Design review of the part built by this model. Coordinates are the model's own, in mm. A direction names the side the tool comes from. Give positions to 0.01 mm unless a question says otherwise; leave off trailing zeros. Write each loop counter-clockwise with the first axis right and the second up, starting at its lowest first coordinate (ties: lowest second). Pieces come first, ordered by that corner, then holes.
```python
from build123d import *
from build123d.topology import SkipClean

# Parameters (mm, degrees)
SKETCH1_R           = 1.1
BOSS_EXTRUDE1_DEPTH = 1.12
SKETCH1_3_W         = 5.75
SKETCH1_3_H         = 5.75
BOSS_EXTRUDE2_DEPTH = 7
SKETCH1_4_W         = 10.8
SKETCH1_4_H         = 10.8
SKETCH1_4_W_2       = 5.75
SKETCH1_4_H_2       = 5.75
BOSS_EXTRUDE3_DEPTH = 5
BOSS_EXTRUDE4_DEPTH = 2
BOSS_EXTRUDE5_START = 0.1
SKETCH1_7_R         = 2
SKETCH1_7_R_2       = 1.1
BOSS_EXTRUDE5_DEPTH = 0.1
CHAMFER1_SIZE       = 1.7
SKETCH3_R           = 2.25
BOSS_EXTRUDE6_DEPTH = 1
BOSS_EXTRUDE6_TAPER = 60
FILLET1_R           = 1.5
SKETCH4_W           = 13
SKETCH4_H           = 4
BOSS_EXTRUDE7_DEPTH = 2.75


with BuildPart() as part:
    # Sketch1 → Boss-Extrude1 (new body)
    with BuildSketch(Plane(origin=(0, 0, 0), x_dir=(1, 0, 0), z_dir=(0, 1, 0))):
        with BuildLine():
            Line((-10.5, -11.931), (10.5, -11.931))
            ThreePointArc((10.5, -11.931), (11.914213562, -11.345213562), (12.5, -9.931))
            Line((12.5, -9.931), (12.5, 9.931))
            ThreePointArc((12.5, 9.931), (11.914213567, 11.345213558), (10.500000012, 11.931))
            Line((10.500000012, 11.931), (-10.5, 11.931))
            ThreePointArc((-10.5, 11.931), (-11.914213562, 11.345213562), (-12.5, 9.931))
            Line((-12.5, 9.931), (-12.5, -9.930999993))
            ThreePointArc((-12.5, -9.930999993), (-11.914213565, -11.34521356), (-10.5, -11.931))
        make_face()
        with Locations(Location((10.5, 2.769, 0), (0, 0, 270))):
            Circle(SKETCH1_R, mode=Mode.SUBTRACT)
        with Locations(Location((10.5, -9.931, 0), (0, 0, 270))):
            Circle(SKETCH1_R, mode=Mode.SUBTRACT)
        with Locations(Location((-10.5, -9.931, 0), (0, 0, 270))):
            Circle(SKETCH1_R, mode=Mode.SUBTRACT)
        with Locations(Location((-10.5, 2.769, 0), (0, 0, 270))):
            Circle(SKETCH1_R, mode=Mode.SUBTRACT)
    extrude(amount=-BOSS_EXTRUDE1_DEPTH)

    # Sketch1_3 → Boss-Extrude2 (add)
    with BuildSketch(Plane(origin=(0, 0, 0), x_dir=(1, 0, 0), z_dir=(0, 1, 0))):
        with Locations((0, 2.769)):
            Rectangle(SKETCH1_3_W, SKETCH1_3_H)
    extrude(amount=BOSS_EXTRUDE2_DEPTH)

    # Sketch1_4 → Boss-Extrude3 (add)
    with BuildSketch(Plane(origin=(0, 0, 0), x_dir=(1, 0, 0), z_dir=(0, 1, 0))):
        with Locations((0, 2.769)):
            Rectangle(SKETCH1_4_W, SKETCH1_4_H)
        with Locations((0, 2.769)):
            Rectangle(SKETCH1_4_W_2, SKETCH1_4_H_2, mode=Mode.SUBTRACT)
    extrude(amount=BOSS_EXTRUDE3_DEPTH)

    # Sketch1_6 → Boss-Extrude4 (add)
    with BuildSketch(Plane(origin=(0, 0, 0), x_dir=(1, 0, 0), z_dir=(0, 1, 0))):
        Polygon((3.5, -2.631), (-2.4, -2.631), (-2.4, -9.931), (6.5, -9.931), (6.5, -5.931), (3.5, -5.931), align=None)
    extrude(amount=BOSS_EXTRUDE4_DEPTH)

    # Sketch1_7 → Boss-Extrude5 (add)
    # profile 1 of 4: a face of its own
    with SkipClean():  # the faces are left unmerged after this step: merging them gives an invalid solid
        with BuildSketch(Plane(origin=(0, 0, 0), x_dir=(1, 0, 0), z_dir=(0, 1, 0)).offset(BOSS_EXTRUDE5_START)):
            with Locations(Location((-10.5, 2.769, 0), (0, 0, 180))):
                Circle(SKETCH1_7_R)
            with Locations(Location((-10.5, 2.769, 0), (0, 0, 270))):
                Circle(SKETCH1_7_R_2, mode=Mode.SUBTRACT)
        # profile 2 of 4: a face of its own
        with BuildSketch(Plane(origin=(0, 0, 0), x_dir=(1, 0, 0), z_dir=(0, 1, 0)).offset(BOSS_EXTRUDE5_START)):
            with Locations(Location((-10.5, -9.931, 0), (0, 0, 270))):
                Circle(SKETCH1_7_R)
            with Locations(Location((-10.5, -9.931, 0), (0, 0, 270))):
                Circle(SKETCH1_7_R_2, mode=Mode.SUBTRACT)
        # profile 3 of 4: a face of its own
        with BuildSketch(Plane(origin=(0, 0, 0), x_dir=(1, 0, 0), z_dir=(0, 1, 0)).offset(BOSS_EXTRUDE5_START)):
            with Locations((10.5, 2.769)):
                Circle(SKETCH1_7_R)
            with Locations(Location((10.5, 2.769, 0), (0, 0, 270))):
                Circle(SKETCH1_7_R_2, mode=Mode.SUBTRACT)
        # profile 4 of 4: a face of its own
        with BuildSketch(Plane(origin=(0, 0, 0), x_dir=(1, 0, 0), z_dir=(0, 1, 0)).offset(BOSS_EXTRUDE5_START)):
            with Locations(Location((10.5, -9.931, 0), (0, 0, 270))):
                Circle(SKETCH1_7_R)
            with Locations(Location((10.5, -9.931, 0), (0, 0, 270))):
                Circle(SKETCH1_7_R_2, mode=Mode.SUBTRACT)
        extrude(amount=-BOSS_EXTRUDE5_DEPTH)

    # Chamfer1
    chamfer1_edges = [part.edges().sort_by_distance(p)[0] for p in [
        (-2.875, 6, -5.644),
        (-2.875, 6, 0.106),
        (2.875, 6, 0.106),
        (2.875, 6, -5.644),
    ]]
    chamfer(chamfer1_edges, length=CHAMFER1_SIZE)

    # Sketch3 → Boss-Extrude6 (add)
    with SkipClean():  # the faces are left unmerged after this step: merging them gives an invalid solid
        with BuildSketch(Plane(origin=(0, 7, 0), x_dir=(1, 0, 0), z_dir=(0, 1, 0))):
            with Locations((0, 2.769)):
                Circle(SKETCH3_R)
        extrude(amount=BOSS_EXTRUDE6_DEPTH, taper=BOSS_EXTRUDE6_TAPER)

    # Fillet1
    fillet1_edges = [part.edges().sort_by_distance(p)[0] for p in [
        (-0.517949192, 8, -2.769),
    ]]
    fillet(fillet1_edges, radius=FILLET1_R)

    # Sketch4 → Boss-Extrude7 (add)
    with SkipClean():  # the faces are left unmerged after this step: merging them gives an invalid solid
        with BuildSketch(Plane.XZ.offset(1.12)):
            with Locations((0, 9.831)):
                Rectangle(SKETCH4_W, SKETCH4_H)
        extrude(amount=BOSS_EXTRUDE7_DEPTH)


solid = part.part
```
(1) Consider section C-C, the plane x = -3.75. Give the boundary of the cut face in (y, z), then the cut area to 3 significant figures.
Resolved:
outline: (-3.87, 7.83) - (-1.12, 7.83) - (-1.12, -11.93) - (0, -11.93) - (0, -8.17) - (5, -8.17) - (5, 2.63) - (0, 2.63) - (0, 11.93) - (-1.12, 11.93) - (-1.12, 11.83) - (-3.87, 11.83) - close
area: 91.7 mm2
(2) Mouldability with a two-part tool opening along Z and no side actions: class faces 5 (the face through (3.5, 1, 4)), 6 (the face through (1, 2, 6)), 7 (the face through (5, 1, 5.931)), 8 (the face through (0.1, -0.6, -11.931)) as pulls with the +Z half, pulls with the -Z half, needs draft (parallel to the pull), parting line crosses it, or undercut.
Resolved:
face 5: undercut
face 6: needs draft
face 7: undercut
face 8: pulls with the -Z half
(3) To check wall thickness, follow L1, parallel to Y at x = -9.25, z = 9; L2, parallel to Z at x = -5, y = 2.25; L3, parallel to X at y = 4.5, z = -1. State the ranges of each line that lie inside material, in increasing order.
Resolved:
L1: y = -1.12 to 0.1
L2: z = -8.17 to 2.63
L3: x = -5.4 to 5.4
(4) Clearance check with flat-ended pins moving along their axes: P1, Ø7, axis at x = -3.5, z = 4, coming from the +Y side; P2, Ø1, axis at x = -3, z = -2.5, coming from the -Y side; P3, Ø4, axis at x = 0.5, y = 3, coming from the +Z side. State where each tip first meets the part, or that it passes through.
Resolved:
P1: stops at y = 5
P2: stops at y = -1.12
P3: stops at z = 9.93
(5) Consider section D-D, the plane x = -9. Give the boundary of the cut face in (y, z), then the cut area to 3 significant figures.
Resolved:
outline: (-1.12, -11.93) - (0, -11.93) - (0, -4.09) - (0.1, -4.09) - (0.1, -1.45) - (0, -1.45) - (0, 8.61) - (0.1, 8.61) - (0.1, 11.25) - (0, 11.25) - (0, 11.93) - (-1.12, 11.93) - close
area: 27.3 mm2
(6) Consider section A-A, the plane z = 4. Give the boundary of the cut face in (x, y).
Resolved:
outline: (-12.5, -1.12) - (12.5, -1.12) - (12.5, 0) - (3.5, 0) - (3.5, 2) - (-2.4, 2) - (-2.4, 0) - (-12.5, 0) - close
(7) Tool access review of faces 1 (the face through (0, 6, -5.644)), 2 (the face through (-2, 5, 0)), 3 (the face through (2.01, 5.99, -4.81)), 4 (the face through (-2.04, 5.99, -4.78)): name each direction out of +Z, -Z, +X, -X, +Y, -Y from which nothing blocks a thin tool from reaching the whole face with its end or side.
Resolved:
face 1: -Z, +X, -X, +Y
face 2: +Y
face 3: -Z, +X, +Y
face 4: -Z, -X, +Y
(8) Consider section B-B, the plane y = 5.5. Give the boundary of the cut face in (x, z) (3 decimals), then the cut area to 3 significant figures.
Resolved:
outline: (-2.875, -3.944) - (-1.175, -5.644) - (1.175, -5.644) - (2.875, -3.944) - (2.875, -1.594) - (1.175, 0.106) - (-1.175, 0.106) - (-2.875, -1.594) - close
area: 27.3 mm2
